Read the model definition and answer for the solid it produces. Units are mm, in the model's axes. A direction names the side the tool comes from. Give positions to 0.01 mm unless a question says otherwise; leave off trailing zeros. Order: outer loops, then holes, each group sorted by start corner. A loop starts at its lowest first (then second) coordinate and runs counter-clockwise, first axis right, second up.
Item 1: Find the intervals of material crossed by line 1 along X through (y, z) = (1.55, -2.5); line 2 along Z through (x, y) = (2, 0.4); line 3 along X through (y, z) = (1.4, -20.5), in increasing order.
Item 2: The mould has two halves that part along X. Classify faces 5 (the face through (26.5, 1, -15)), 6 (the face through (18, 1, -3)), 7 (the face through (13, 0, -15)), 8 (the face through (0, 1, -3)): +X half, -X half, draft (parallel to the pull), parting line (faces both ways), or undercut.
Item 3: A cutting plane is placed at B-B (z = -20.5). Write down the section's boundary in (x, y), plus the area to 3 significant figures.
Item 4: A cutting plane is placed at C-C (x = 10.5). Write down the section's boundary in (y, z).
Item 5: Given pin 1 Ø1.5 at (x, y) = (1, 2) entering from -Z; pin 2 Ø0.9 at (x, y) = (17.5, 1) entering from +Z, each flat-ended and moving along its own axis, determine where each tip first touches the part or whether it passes through.
Item 6: Which of the six approach directions +Z, -Z, +X, -X, +Y, -Y give full straight-line access (tool end or side, diameter ignored) to faces 1 (the face through (3, 1, -24)), 2 (the face through (23.5, 1, -24)), 3 (the face through (15.5, 1, -2)), 4 (the face through (25, 1, -12))?
Item 7: A cutting plane is placed at A-A (y = 2.2). Write down the section's boundary in (x, z), plus the area to 3 significant figures.
from build123d import *

# Parameters (mm, degrees)
PAREDELADO2_DEPTH = 3


with BuildPart() as part:
    # ParedeLado2Esboco → ParedeLado2 (new body)
    with BuildSketch(Plane(origin=(0, 0, 0), x_dir=(1, 0, 0), z_dir=(0, 1, 0))):
        Polygon((0, 0), (0, 6), (3, 6), (3, 12), (0, 12), (0, 18), (3, 18), (3, 30), (23.5, 30), (23.5, 18), (26.5, 18), (26.5, 12), (23.5, 12), (23.5, 6), (26.5, 6), (26.5, 0), (20.5, 0), (20.5, 3), (15.5, 3), (15.5, 0), (11, 0), (11, 3), (6, 3), (6, 0), align=None)
    extrude(amount=PAREDELADO2_DEPTH)


solid = part.part
Response values:
1. line 1: x = 0 to 6, 11 to 15.5, 20.5 to 26.5
1. line 2: z = -18 to -12, -6 to 0
1. line 3: x = 3 to 23.5
2. face 5: +X half
2. face 6: undercut
2. face 7: draft
2. face 8: -X half
3. outline: (3, 0) - (23.5, 0) - (23.5, 3) - (3, 3) - close
3. area: 61.5 mm2
4. outline: (0, -30) - (3, -30) - (3, -3) - (0, -3) - close
5. pin 1: stops at z = -18
5. pin 2: stops at z = -3
6. face 1: -Z, -X, +Y, -Y
6. face 2: -Z, +X, +Y, -Y
6. face 3: +Z, +Y, -Y
6. face 4: +X, +Y, -Y
7. outline: (0, -18) - (3, -18) - (3, -30) - (23.5, -30) - (23.5, -18) - (26.5, -18) - (26.5, -12) - (23.5, -12) - (23.5, -6) - (26.5, -6) - (26.5, 0) - (20.5, 0) - (20.5, -3) - (15.5, -3) - (15.5, 0) - (11, 0) - (11, -3) - (6, -3) - (6, 0) - (0, 0) - (0, -6) - (3, -6) - (3, -12) - (0, -12) - close
7. area: 657 mm2
